```python
from build123d import *

# Parameters (mm, degrees)
F0_W     = 55
F0_H     = 48
F1_DEPTH = 2
F0_W_2   = 58.2
F0_H_2   = 51.2
F2_DEPTH = 42
F4_DEPTH = 4


with BuildPart() as f1:
    # F0 (on Top) → F1 (new body)
    with BuildSketch(Plane.XY):
        Rectangle(F0_W, F0_H)
    extrude(amount=F1_DEPTH)

    # F0 (on Top) → F2 (join)
    with BuildSketch(Plane.XY):
        Rectangle(F0_W_2, F0_H_2)
        Rectangle(F0_W, F0_H, mode=Mode.SUBTRACT)
    extrude(amount=F2_DEPTH)

    # F3 (on face) → F4 (cut)
    with BuildSketch(Plane.YZ.offset(29.1)):
        with BuildLine():
            ThreePointArc((-10.778551, 20.545242), (6.221449, 37.545242), (23.221449, 20.545242))
            Line((23.221449, 20.545242), (23.221449, 42))
            Line((23.221449, 42), (-10.778551, 42))
            Line((-10.778551, 42), (-10.778551, 20.545242))
        make_face()
        with BuildLine():
            ThreePointArc((-10.778551, 20.545242), (6.221449, 3.545242), (23.221449, 20.545242))
            ThreePointArc((23.221449, 20.545242), (6.221449, 37.545242), (-10.778551, 20.545242))
        make_face()
    extrude(amount=-F4_DEPTH, mode=Mode.SUBTRACT)


solid = f1.part
```
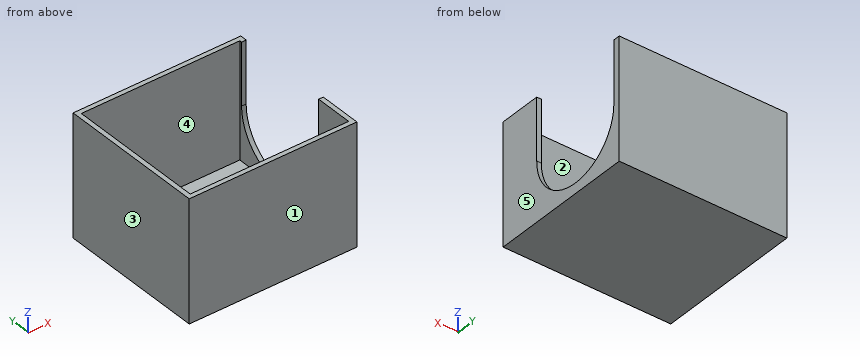
Build history of the part. All positions in model axes, mm. Face numbers are marked on the shaded views. A direction names the side the tool comes from. Round coordinates to 2 decimals unless told otherwise and drop trailing zeros. Loops run counter-clockwise (first coordinate to the right, second up) from the corner with the lowest first, then second, coordinate; pieces in that order, holes last. Notation, with made-up numbers: M 58,-40 L 91,-40 A7 cw 91,-27 Z; hole C -30,38.25 d4. An arc over 180 degrees is marked long. Answer as CSV lines item,"result".
1. Two-plate mould, pull along X, no slides. Class the marked faces 1, 2 and 3: released by +X, released by -X, zero draft, split by the parting line, or undercut.
Resolved:
face 1,"zero draft"
face 2,"undercut"
face 3,"released by -X"
2. Wall check: probe 1 along Y at (x, z) = (12.5, 12.5); probe 2 along X at (y, z) = (-21, 13.5); probe 3 along X at (y, z) = (8.5, 10.5). Give the ranges that are in metal, low to high. Write a range as [from, to].
Resolved:
probe 1,"y = [-25.6, -24], [24, 25.6]"
probe 2,"x = [-29.1, -27.5], [27.5, 29.1]"
probe 3,"x = [-29.1, -27.5]"
3. Cut at A-A on x = 20.5. Write the cut outline in (y, z).
Resolved:
outline,"M -25.6,0 L 25.6,0 L 25.6,42 L 24,42 L 24,2 L -24,2 L -24,42 L -25.6,42 Z"
4. 3-axis set-ups, long thin cutter, end or side, ignore diameter. For the marked faces 4 and 5: which of +Z, -Z, +X, -X, +Y, -Y reach the whole face in a straight line?
Resolved:
face 4,"+Z"
face 5,"+Z, -Z, +X, +Y, -Y"
5. Cut at C-C on z = 35.5. Write the cut outline in (x, y).
Resolved:
outline,"M -29.1,-25.6 L 29.1,-25.6 L 29.1,-10.78 L 27.5,-10.78 L 27.5,-24 L -27.5,-24 L -27.5,24 L 27.5,24 L 27.5,23.22 L 29.1,23.22 L 29.1,25.6 L -29.1,25.6 Z"
6. Cut at B-B on y = -17.5. Write the cut outline in (x, z).
Resolved:
outline,"M -29.1,0 L 29.1,0 L 29.1,42 L 27.5,42 L 27.5,2 L -27.5,2 L -27.5,42 L -29.1,42 Z"
7. Flat gauge pins, fed straight in: P1, Ø3, axis at y = -5.5, z = 17.5, coming from the +X side; P2, Ø24, axis at x = 2.5, y = -4.5, coming from the +Z side. Where does each tip first touch, or does it go through?
Resolved:
P1,"stops at x = -27.5"
P2,"stops at z = 2"
8. Cut at D-D on z = 14. Write the cut outline in (x, y).
Resolved:
outline,"M -29.1,-25.6 L 29.1,-25.6 L 29.1,-9.47 L 27.5,-9.47 L 27.5,-24 L -27.5,-24 L -27.5,24 L 27.5,24 L 27.5,21.91 L 29.1,21.91 L 29.1,25.6 L -29.1,25.6 Z"
